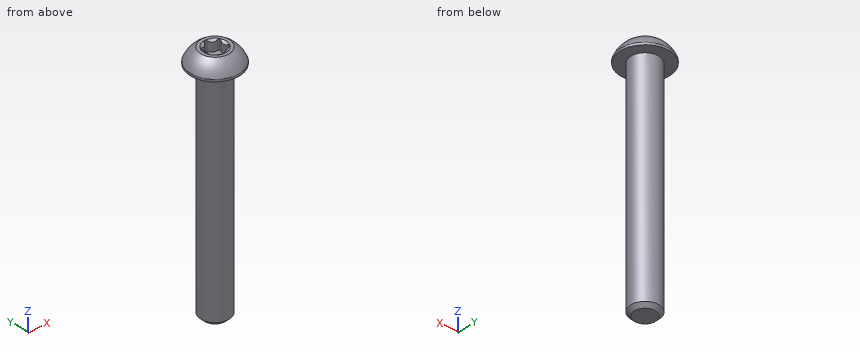
```python
from build123d import *

# Parameters (mm, degrees)
CUT_EXTRUDE1_DEPTH = 2.34696
CIRPATTERN1_COUNT  = 6


with BuildPart() as part:
    # Sketch3 → Revolve1 (revolve)
    with BuildSketch(Plane(origin=(0, 0, 0), x_dir=(0, 0, -1), z_dir=(1, 0, 0))):
        with BuildLine():
            Line((2.84988, 5.5499), (3.3528, 5.5499))
            Line((3.3528, 5.5499), (3.3528, 3.175))
            Line((3.3528, 3.175), (53.337781533, 3.175))
            Line((53.337781533, 3.175), (54.1528, 2.359981533))
            Line((54.1528, 2.359981533), (54.1528, 0))
            Line((54.1528, 0), (0, 0))
            Line((0, 0), (0, 3.175))
            ThreePointArc((0, 3.175), (1.235921075, 4.58927271), (2.84988, 5.5499))
        make_face()
    revolve(axis=Axis((0, 0, -54.1528), (0, 0, 1)))

    # Sketch4 → Cut-Extrude1 (cut)
    with BuildSketch(Plane.XY):
        with BuildLine():
            Line((0, 0), (-2.199704526, -1.27))
            ThreePointArc((-2.199704526, -1.27), (-2.242070202, -1.100823133), (-2.188690187, -0.934792301))
            ThreePointArc((-2.188690187, -0.934792301), (-1.905, 0), (-2.188690187, 0.934792301))
            ThreePointArc((-2.188690187, 0.934792301), (-2.242070202, 1.100823133), (-2.199704526, 1.27))
            Line((-2.199704526, 1.27), (0, 0))
        make_face()
    cut_extrude1 = extrude(amount=-CUT_EXTRUDE1_DEPTH, mode=Mode.SUBTRACT)

    # CirPattern1: Cut-Extrude1 ×6 about axis
    cirpattern1_axis = Axis((0, 0, -54.1528), (0, 0, 1))
    for i in range(1, CIRPATTERN1_COUNT):
        add(cut_extrude1.rotate(cirpattern1_axis, i * 360 / CIRPATTERN1_COUNT), mode=Mode.SUBTRACT)

    # Cut-Extrude2 cone 1 section (through the dimple's axis) → Cut-Extrude2 (revolve, cut)
    with BuildSketch(Plane(origin=(0, 0, 0), x_dir=(0, -1, 0), z_dir=(1, 0, 0))):
        Polygon((0, 0), (2.54, 0), (0, 1.466469684), align=None)
    revolve(axis=Axis((0, 0, 0), (0, 0, -1)), mode=Mode.SUBTRACT)


solid = part.part
```
Geometry check sheet. Reference: the model listing, model coordinates, mm. Coordinates: 2 decimals unless noted, no trailing zeros. Order: outer loops, then holes, each group sorted by start corner. A loop starts at its lowest first (then second) coordinate and runs counter-clockwise, first axis right, second up. Notation, with made-up numbers: (39.25, 77.5) - (51.25, 77.5) arc R30 ccw to (51.25, 105.5) - close; hole circle Ø9 at (-30, 3.25). An arc over 180 degrees is marked (long way). Use one line per item in the form item = value.
1. Section check B-B (z = -51). Record the boundary of the cut face in (x, y) (3 decimals), then the cut area to 3 significant figures.
Here are the results:
outline = circle Ø6.35 at (0, 0)
area = 31.7 mm²
2. Section check A-A (y = 0). Record the boundary of the cut face in (x, z) (3 decimals).
Here are the results:
outline = (-5.55, -3.353) - (-3.175, -3.353) - (-3.175, -53.338) - (-2.36, -54.153) - (2.36, -54.153) - (3.175, -53.338) - (3.175, -3.353) - (5.55, -3.353) - (5.55, -2.85) arc R5.974 ccw to (3.175, 0) - (2.54, 0) - (1.905, -0.367) - (1.905, -2.347) - (-1.905, -2.347) - (-1.905, -0.367) - (-2.54, 0) - (-3.175, 0) arc R5.974 ccw to (-5.55, -2.85) - close
3. Scan lines: line 1 (Z direction, x = -0.5, y = 1.5); line 2 (X direction, y = 2.25, z = -4); line 3 (Z direction, x = 1.5, y = -4.5). Record each from-to range of solid material in increasing order.
Here are the results:
line_1 = -54.15 to -2.35
line_2 = -2.24 to 2.24
line_3 = -3.35 to -1.43
4. Gauge pin test, flat ends, axial feed: pin 1 (2 mm diameter, centred on x = 1, y = -0.5, fed in from +Z); pin 2 (4 mm diameter, centred on x = 3.5, z = -15.5, fed in from +Y); pin 3 (4 mm diameter, centred on y = 0, z = -35, fed in from +X) (3 decimals). Record the tip position at first contact, or that the pin passes through.
Here are the results:
pin_1 = -0.27
pin_2 = 2.8
pin_3 = 3.175
5. Section check C-C (x = -4.5). Record the boundary of the cut face in (y, z), then the cut area to 3 significant figures.
Here are the results:
outline = (-3.25, -3.35) - (3.25, -3.35) - (3.25, -2.85) arc R3.93 ccw to (-3.25, -2.85) - close
area = 11.1 mm²
6. Section check D-D (x = 4.75). Record the boundary of the cut face in (y, z).
Here are the results:
outline = (-2.87, -3.35) - (2.87, -3.35) - (2.87, -2.85) arc R3.62 ccw to (-2.87, -2.85) - close
